Input: part model. Units: mm. Frame: model coordinates. Give positions to 0.01 mm unless a question says otherwise; leave off trailing zeros. Loops run counter-clockwise (first coordinate to the right, second up) from the corner with the lowest first, then second, coordinate; pieces in that order, holes last. Notation, with made-up numbers: M 67.25,-27.5 L 88.25,-27.5 A17 cw 88.25,-6.5 Z; hole C 86,44 d2. An arc over 180 degrees is marked long. Answer as a JSON object with one key per item and string values. Group by question number.
1) Ray query, L1, parallel to Y at x = -42, z = 2.7; L2, parallel to X at y = -41.5, z = 2.95. Return the intervals inside material, ascending.
2) Section query B-B on x = -45.5. Return loops of the section in (y, z).
3) First-contact query: P1, Ø1.5, axis at x = -7.5, y = 119, coming from the -Z side. Flat tip, straight axial feed; report the tip coordinate or a pass-through.
4) Section query A-A on y = -37.5. Return loops of the section in (x, z), plus the area to 3 significant figures.
from build123d import *

# Parameters (mm, degrees)
ESQUISSE1_W             = 150
ESQUISSE1_H             = 355
BOSS_EXTRU_1_DEPTH      = 5
ESQUISSE2_R             = 6
ENL_V_MAT_EXTRU_1_DEPTH = 20
ESQUISSE3_R             = 1.5
ENL_V_MAT_EXTRU_2_DEPTH = 2.25


with BuildPart() as part:
    # Esquisse1 → Boss.-Extru.1 (new body)
    with BuildSketch(Plane.XY):
        Rectangle(ESQUISSE1_W, ESQUISSE1_H)
    extrude(amount=BOSS_EXTRU_1_DEPTH)

    # Esquisse2 → Enlèv. mat.-Extru.1 (cut)
    with BuildSketch(Plane.XY.offset(5)):
        with Locations((-45.5, 78.5)):
            Circle(ESQUISSE2_R)
        with Locations((-45.5, -37.5)):
            Circle(ESQUISSE2_R)
    extrude(amount=-ENL_V_MAT_EXTRU_1_DEPTH, mode=Mode.SUBTRACT)

    # Esquisse3 → Enlèv. mat.-Extru.2 (cut)
    with BuildSketch(Plane(origin=(0, 0, 0), x_dir=(-1, 0, 0), z_dir=(0, 0, -1))):
        with Locations((1.188690161, 154.472601824)):
            Circle(ESQUISSE3_R)
        with Locations((51.906289441, 163.445482985)):
            Circle(ESQUISSE3_R)
        with Locations((7.529151507, 118.554842214)):
            Circle(ESQUISSE3_R)
        with Locations((58.246291945, 127.500325199)):
            Circle(ESQUISSE3_R)
        with Locations((7.529151507, -77.584842214)):
            Circle(ESQUISSE3_R)
        with Locations((58.246291945, -86.530325199)):
            Circle(ESQUISSE3_R)
        with Locations((1.188690161, -113.502601824)):
            Circle(ESQUISSE3_R)
        with Locations((51.906289441, -122.475482985)):
            Circle(ESQUISSE3_R)
    extrude(amount=-ENL_V_MAT_EXTRU_2_DEPTH, mode=Mode.SUBTRACT)


solid = part.part
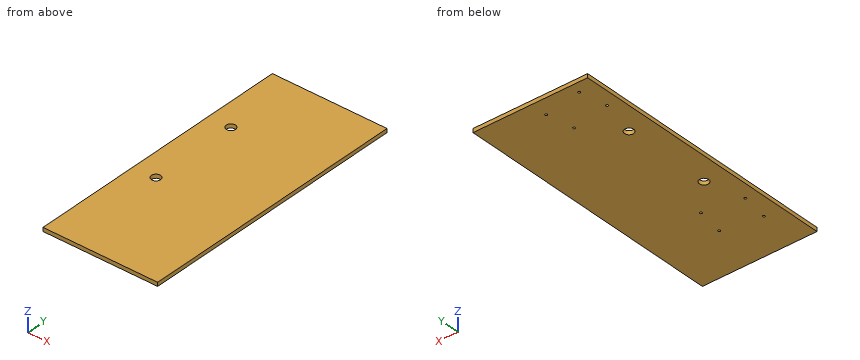
Output:
{
 "1": {"L1": "y = -177.5 to -42.37, -32.63 to 73.63, 83.37 to 177.5", "L2": "x = -75 to -49.97, -41.03 to 75"},
 "2": {"outline": "M -177.5,0 L -43.5,0 L -43.5,5 L -177.5,5 Z; M -31.5,0 L 72.5,0 L 72.5,5 L -31.5,5 Z; M 84.5,0 L 177.5,0 L 177.5,5 L 84.5,5 Z"},
 "3": {"P1": "stops at z = 2.25"},
 "4": {"outline": "M -75,0 L -51.5,0 L -51.5,5 L -75,5 Z; M -39.5,0 L 75,0 L 75,5 L -39.5,5 Z", "area": "690 mm^2"}
}
